```python
from build123d import *

# Parameters (mm, degrees)
F1_DEPTH = 4
F2_R     = 5
F2_R_2   = 3.4
F2_R_3   = 5.5
F3_DEPTH = 8
F4_R     = 4


with BuildPart() as f1:
    # F0 (on Front) → F1 (new body, symmetric)
    with BuildSketch(Plane.XZ):
        Polygon((500, -92), (440, 92), (-440, 92), (-500, -92), (-440, -92), (440, -92), align=None)
    extrude(amount=F1_DEPTH, both=True)

    # F2 (on face) → F3 (cut)
    with BuildSketch(Plane.XZ.offset(4)):
        with Locations((429, 5)):
            Circle(F2_R)
        with Locations((420, 72)):
            Circle(F2_R_2)
        with Locations((-420, 72)):
            Circle(F2_R_2)
        with Locations((-429, 5)):
            Circle(F2_R)
        with Locations((0, -2)):
            Circle(F2_R_3)
    extrude(amount=-F3_DEPTH, mode=Mode.SUBTRACT)

    # F4
    f4_edges = [f1.edges().sort_by_distance(p)[0] for p in [
        (500, 0, -92),
        (-500, 0, -92),
        (440, 0, 92),
        (-440, 0, 92),
    ]]
    fillet(f4_edges, radius=F4_R)


solid = f1.part
```
Geometry check sheet. Reference: the model listing, model coordinates, mm. Round coordinates to 2 decimals unless told otherwise and drop trailing zeros. Write each loop counter-clockwise with the first axis right and the second up, starting at its lowest first coordinate (ties: lowest second). Pieces come first, ordered by that corner, then holes. Notation, with made-up numbers: (24, -32.5) - (71, -32.5) arc R13 cw to (71, -26.5) - close; hole circle Ø4 at (-11, 43.5). An arc over 180 degrees is marked (long way). Write each question's results on one line, items separated by ' | '.
(1) Sectioned sample at C-C, the plane z = -36.5. Enter the section's corners in (x, y).
Computed:
outline: (-481.9, -4) - (481.9, -4) - (481.9, 4) - (-481.9, 4) - close
(2) Sectioned sample at A-A, the plane y = -0.5. Enter the section's corners in (x, z).
Computed:
outline: (-498.29, -86.76) arc R4 ccw to (-494.49, -92) - (494.49, -92) arc R4 ccw to (498.29, -86.76) - (440.9, 89.24) arc R4 ccw to (437.1, 92) - (-437.1, 92) arc R4 ccw to (-440.9, 89.24) - close; hole circle Ø10 at (-429, 5); hole circle Ø6.8 at (-420, 72); hole circle Ø11 at (0, -2); hole circle Ø6.8 at (420, 72); hole circle Ø10 at (429, 5)
(3) Sectioned sample at B-B, the plane z = 38. Enter the section's corners in (x, y).
Computed:
outline: (-457.61, -4) - (457.61, -4) - (457.61, 4) - (-457.61, 4) - close
(4) Depth check by flat-ended pin: pin 1 Ø3 at (y, z) = (1, 23.5) entering from +X; pin 2 Ø1.5 at (y, z) = (-3, 38) entering from +X; pin 3 Ø1 at (y, z) = (0, -9) entering from +X; pin 4 Ø4 at (x, z) = (420, 72) entering from -Y. Enter the tip coordinate at first touch or a pass-through.
Computed:
pin 1: stops at x = 462.83 | pin 2: stops at x = 457.85 | pin 3: stops at x = 473.1 | pin 4: passes through
(5) Thickness scan on probe 1 along Z at (x, y) = (429, 2); probe 2 along Z at (x, y) = (-420, -0.5); probe 3 along X at (y, z) = (-2.5, -3). Record the ranges inside material, lowest first. Write a range as from..to.
Computed:
probe 1: z = -92..0, 10..92 | probe 2: z = -92..68.6, 75.4..92 | probe 3: x = -470.98..-5.41, 5.41..470.98
